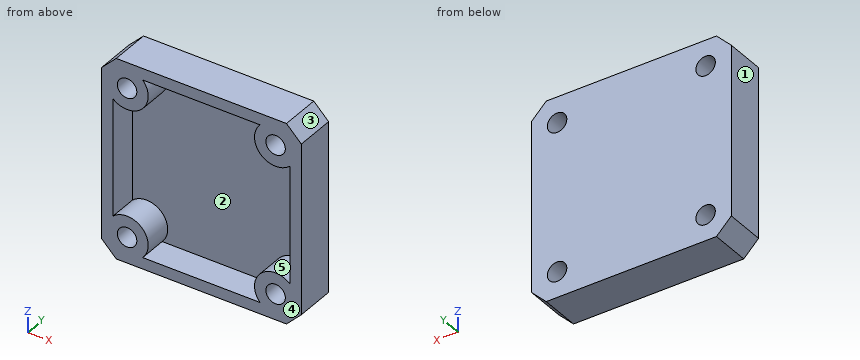
Autodesk Inventor part; units mm, degrees
ref_plane "YZ Plane" through (0, 0, 0) normal (1, 0, 0) x (0, 1, 0)
ref_plane "XZ Plane" through (0, 0, 0) normal (0, 1, 0) x (-1, 0, 0)
ref_plane "XY Plane" through (0, 0, 0) normal (0, 0, 1) x (1, 0, 0)
sketch "Sketch1" plane through (0, 0, 0) normal (0, 1, 0) x (-1, 0, 0)
  line L0 (-17.5, 17.5) -> (17.5, 17.5)
  line L1 (17.5, 17.5) -> (17.5, -17.5)
  line L2 (17.5, -17.5) -> (-17.5, -17.5)
  line L3 (-17.5, -17.5) -> (-17.5, 17.5)
  line L4 (-17.5, 17.5) -> (17.5, -17.5) construction
  line L5 (17.5, 17.5) -> (-17.5, -17.5) construction
  line L6 (-13, -13) -> (13, -13) construction
  line L7 (13, -13) -> (13, 13) construction
  line L8 (13, 13) -> (-13, 13) construction
  line L9 (-13, 13) -> (-13, -13) construction
  line L10 (-13, -13) -> (13, 13) construction
  line L11 (13, -13) -> (-13, 13) construction
  circle A0 centre (13, 13) radius 1.7
  circle A1 centre (13, -13) radius 1.7
  circle A2 centre (-13, -13) radius 1.7
  circle A3 centre (-13, 13) radius 1.7
  point P0 (0, 0)
  dimension "d0" = 35
  dimension "d1" = 35
  dimension "d2" = 3.4
  dimension "d3" = 3.4
  dimension "d4" = 3.4
  dimension "d5" = 3.4
  dimension "d6" = 26
  dimension "d7" = 26
extrude "Extrusion1" add sketch "Sketch1" along normal blind 7
chamfer "Chamfer1" distance 2.6 angle 45 4 edges at (17.5, 3.5, 17.5) (-17.5, 3.5, 17.5) (17.5, 3.5, -17.5) (-17.5, 3.5, -17.5)
shell "Shell2" thickness 2 removed faces 1 at (-3.9092, 0, 3.9576)
equation "\"d1\" = d0"
equation "\"d3\" = d2"
equation "\"d4\" = d2"
equation "\"d5\" = d2"
properties part number "PCB_Spacer"
Design review of the part built by this model. Coordinates are the model's own, in mm. Face numbers are marked on the shaded views. A direction names the side the tool comes from. Give positions to 0.01 mm unless a question says otherwise; leave off trailing zeros. Order: outer loops, then holes, each group sorted by start corner. A loop starts at its lowest first (then second) coordinate and runs counter-clockwise, first axis right, second up. Notation, with made-up numbers: (7.5, -15.75) -> (50.5, -15.75) arc R8 ccw to (50.5, -3.75) -> close; hole circle Ø3 at (77.5, -24). An arc over 180 degrees is marked (long way). Write each question's results on one line, items separated by ' | '. Start each with the question number.
Q1. Add section D-D on y = 1.5. Give the boundary of the cut face in (x, z).
Q2. Machinability: for the marked faces 1 and 2, which of the approach directions +Z, -Z, +X, -X, +Y, -Y give a long, thin tool a straight path to every point of the face, cutting with its end or side? Answer none if there is none.
Q3. Add section B-B on y = 5.5. Give the boundary of the cut face in (x, z).
Q4. Wall thickness on L1, parallel to Z at x = 13, y = 1.5; L2, parallel to X at y = 4, z = -1.5; L3, parallel to Z at x = 13, y = 5.5: over which ranges is each line inside the solid? List them lowest first. Write a range as from..to.
Q5. Add section A-A on x = 13. Give the boundary of the cut face in (y, z).
Q6. For pin 1 (2 mm diameter, centred on x = 13, z = 13, fed in from -Y); pin 2 (4 mm diameter, centred on x = -1, z = 3, fed in from -Y), all flat-tipped, find the tip position at first contact; note any pin that passes through.
Q7. Add section C-C on z = -13. Give the boundary of the cut face in (x, y), and give its area (3 significant figures).
Q8. Mouldability with a two-part tool opening along Z and no side actions: class the marked faces 3, 4 and 5 as +Z half, -Z half, draft (parallel to the pull), parting line (faces both ways), or undercut.
Found:
1) outline: (-17.5, -14.9) -> (-14.9, -17.5) -> (14.9, -17.5) -> (17.5, -14.9) -> (17.5, 14.9) -> (14.9, 17.5) -> (-14.9, 17.5) -> (-17.5, 14.9) -> close; hole (-15.5, -10.27) arc R3.7 cw to (-10.27, -15.5) -> (10.27, -15.5) arc R3.7 cw to (15.5, -10.27) -> (15.5, 10.27) arc R3.7 cw to (10.27, 15.5) -> (-10.27, 15.5) arc R3.7 cw to (-15.5, 10.27) -> close; hole circle Ø3.4 at (-13, -13); hole circle Ø3.4 at (-13, 13); hole circle Ø3.4 at (13, -13); hole circle Ø3.4 at (13, 13)
2) face 1: +Z, -Z, -X, +Y, -Y | face 2: -Y
3) outline: (-17.5, -14.9) -> (-14.9, -17.5) -> (14.9, -17.5) -> (17.5, -14.9) -> (17.5, 14.9) -> (14.9, 17.5) -> (-14.9, 17.5) -> (-17.5, 14.9) -> close; hole circle Ø3.4 at (-13, -13); hole circle Ø3.4 at (-13, 13); hole circle Ø3.4 at (13, -13); hole circle Ø3.4 at (13, 13)
4) L1: z = -17.5..-14.7, -11.3..-9.3, 9.3..11.3, 14.7..17.5 | L2: x = -17.5..-15.5, 15.5..17.5 | L3: z = -17.5..-14.7, -11.3..11.3, 14.7..17.5
5) outline: (0, -17.5) -> (7, -17.5) -> (7, -14.7) -> (0, -14.7) -> close; (0, -11.3) -> (7, -11.3) -> (7, 11.3) -> (0, 11.3) -> (0, 9.3) -> (5, 9.3) -> (5, -9.3) -> (0, -9.3) -> close; (0, 14.7) -> (7, 14.7) -> (7, 17.5) -> (0, 17.5) -> close
6) pin 1: passes through | pin 2: stops at y = 5
7) outline: (-17.5, 0) -> (-14.7, 0) -> (-14.7, 7) -> (-17.5, 7) -> close; (-11.3, 0) -> (-9.3, 0) -> (-9.3, 5) -> (9.3, 5) -> (9.3, 0) -> (11.3, 0) -> (11.3, 7) -> (-11.3, 7) -> close; (14.7, 0) -> (17.5, 0) -> (17.5, 7) -> (14.7, 7) -> close | area: 104 mm2
8) face 3: +Z half | face 4: draft | face 5: undercut
